Geometry check sheet. Reference: the model listing, model coordinates, mm. Coordinates: 2 decimals unless noted, no trailing zeros. Order: outer loops, then holes, each group sorted by start corner. A loop starts at its lowest first (then second) coordinate and runs counter-clockwise, first axis right, second up. Notation, with made-up numbers: (89.25, -6) - (96.25, -6) arc R13 cw to (96.25, 9) - close; hole circle Ø4 at (-14, 50.25). An arc over 180 degrees is marked (long way). Return JSON: item names as keys, results as strings. Group by question number.
Item 1: Scan lines: probe 1 along Y at (x, z) = (34, -25.1); probe 2 along Y at (x, z) = (104, -25.55); probe 3 along X at (y, z) = (-13, -25.75). Record each from-to range of solid material in increasing order.
Item 2: Draft check along X on faces 1 (the cylindrical face through (-1, 0, -24)), 2 (the cylindrical face through (2.386, 11.425, -24.028)), 3 (the flat face through (51, -30, -24)). Enter one of: pulls with the +X half, pulls with the -X half, needs draft (parallel to the pull), parting line crosses it, or undercut.
Item 3: Section check A-A on y = 0. Enter the section's corners in (x, z).
Item 4: Gauge pin test, flat ends, axial feed: pin 1 (1 mm diameter, centred on x = 9, z = -22.5, fed in from +Y); pin 2 (10.5 mm diameter, centred on x = 16, y = 34, fed in from +Z). Record the tip position at first contact, or that the pin passes through.
Item 5: Section check B-B on z = -25.3. Give the number of separate pieces and of enclosed holes in the cut face, then the cut area to 3 significant figures.
from build123d import *

# Parameters (mm, degrees)
CYLINDER1946_R     = 17
CYLINDER1946_DEPTH = 160
CYLINDER1910_R     = 1.5
CYLINDER1910_DEPTH = 100
CYLINDER1943_R     = 1.5
CYLINDER1943_DEPTH = 100
CYLINDER1944_R     = 1.5
CYLINDER1944_DEPTH = 32
CYLINDER1903_R     = 1.5
CYLINDER1903_DEPTH = 32
BOX555_W           = 200
BOX555_H           = 100
BOX555_DEPTH       = 100
BOX556_W           = 200
BOX556_H           = 100
BOX556_DEPTH       = 100
CYLINDER1907_R     = 4
CYLINDER1907_DEPTH = 100
CYLINDER1908_R     = 4
CYLINDER1908_DEPTH = 100
CYLINDER1912_R     = 4
CYLINDER1912_DEPTH = 100
CYLINDER1913_R     = 4
CYLINDER1913_DEPTH = 100
CYLINDER1914_R     = 4
CYLINDER1914_DEPTH = 100
CYLINDER1901_R     = 4
CYLINDER1901_DEPTH = 100
CYLINDER1902_R     = 4
CYLINDER1902_DEPTH = 100
CYLINDER1919_R     = 4
CYLINDER1919_DEPTH = 100
CYLINDER1927_R     = 1.5
CYLINDER1927_DEPTH = 100
CYLINDER1926_R     = 1.5
CYLINDER1926_DEPTH = 100
CYLINDER1891_R     = 1.5
CYLINDER1891_DEPTH = 100
CYLINDER1894_R     = 1.5
CYLINDER1894_DEPTH = 100
CYLINDER1917_R     = 1.5
CYLINDER1917_DEPTH = 100
CYLINDER1898_R     = 1.5
CYLINDER1898_DEPTH = 100
CYLINDER1920_R     = 1.5
CYLINDER1920_DEPTH = 100
CYLINDER1924_R     = 1.5
CYLINDER1924_DEPTH = 100
CYLINDER1925_R     = 59
CYLINDER1925_DEPTH = 4
FILLET029_R        = 8
FILLET027_R        = 8


with BuildPart() as obj1:
    # Cylinder1946 → Cylinder1946 (new body)
    with BuildSketch(Plane(origin=(-18, 0, -60), x_dir=(1, 0, 0), z_dir=(0, 0, 1))):
        Circle(CYLINDER1946_R)
    extrude(amount=CYLINDER1946_DEPTH)


with BuildPart() as obj2:
    # Cylinder1910 → Cylinder1910 (new body)
    with BuildSketch(Plane(origin=(14, 0, -60), x_dir=(1, 0, 0), z_dir=(0, 0, 1))):
        Circle(CYLINDER1910_R)
    extrude(amount=CYLINDER1910_DEPTH)


with BuildPart() as obj3:
    # Cylinder1943 → Cylinder1943 (new body)
    with BuildSketch(Plane(origin=(90, 0, -60), x_dir=(1, 0, 0), z_dir=(0, 0, 1))):
        Circle(CYLINDER1943_R)
    extrude(amount=CYLINDER1943_DEPTH)

    # Compound988: union obj2
    add(obj2.part)


with BuildPart() as obj4:
    # Cylinder1944 → Cylinder1944 (new body)
    with BuildSketch(Plane(origin=(78, 41, -42), x_dir=(1, 0, 0), z_dir=(0, 0, 1))):
        Circle(CYLINDER1944_R)
    extrude(amount=CYLINDER1944_DEPTH)


with BuildPart() as compound991:
    # Cylinder1903 → Cylinder1903 (new body)
    with BuildSketch(Plane(origin=(26, 41, -42), x_dir=(1, 0, 0), z_dir=(0, 0, 1))):
        Circle(CYLINDER1903_R)
    extrude(amount=CYLINDER1903_DEPTH)

    # Compound991: union obj4
    add(obj4.part)


with BuildPart() as krychle555:
    # Box555 → Box555 (new body)
    with BuildSketch(Plane(origin=(-60, 44, -90), x_dir=(1, 0, 0), z_dir=(0, 0, 1))):
        with Locations((100, 50)):
            Rectangle(BOX555_W, BOX555_H)
    extrude(amount=BOX555_DEPTH)


with BuildPart() as krychle556:
    # Box556 → Box556 (new body)
    with BuildSketch(Plane(origin=(-60, -130, -90), x_dir=(1, 0, 0), z_dir=(0, 0, 1))):
        with Locations((100, 50)):
            Rectangle(BOX556_W, BOX556_H)
    extrude(amount=BOX556_DEPTH)


with BuildPart() as obj5:
    # Cylinder1907 → Cylinder1907 (new body)
    with BuildSketch(Plane(origin=(-16, 34, -90), x_dir=(1, 0, 0), z_dir=(0, 0, 1))):
        Circle(CYLINDER1907_R)
    extrude(amount=CYLINDER1907_DEPTH)


with BuildPart() as obj6:
    # Cylinder1908 → Cylinder1908 (new body)
    with BuildSketch(Plane(origin=(-16, -34, -90), x_dir=(1, 0, 0), z_dir=(0, 0, 1))):
        Circle(CYLINDER1908_R)
    extrude(amount=CYLINDER1908_DEPTH)


with BuildPart() as obj7:
    # Cylinder1912 → Cylinder1912 (new body)
    with BuildSketch(Plane(origin=(34, -16, -90), x_dir=(1, 0, 0), z_dir=(0, 0, 1))):
        Circle(CYLINDER1912_R)
    extrude(amount=CYLINDER1912_DEPTH)


with BuildPart() as obj8:
    # Cylinder1913 → Cylinder1913 (new body)
    with BuildSketch(Plane(origin=(16, 34, -90), x_dir=(1, 0, 0), z_dir=(0, 0, 1))):
        Circle(CYLINDER1913_R)
    extrude(amount=CYLINDER1913_DEPTH)


with BuildPart() as obj9:
    # Cylinder1914 → Cylinder1914 (new body)
    with BuildSketch(Plane(origin=(16, -34, -90), x_dir=(1, 0, 0), z_dir=(0, 0, 1))):
        Circle(CYLINDER1914_R)
    extrude(amount=CYLINDER1914_DEPTH)


with BuildPart() as obj10:
    # Cylinder1901 → Cylinder1901 (new body)
    with BuildSketch(Plane(origin=(-34, 16, -90), x_dir=(1, 0, 0), z_dir=(0, 0, 1))):
        Circle(CYLINDER1901_R)
    extrude(amount=CYLINDER1901_DEPTH)


with BuildPart() as obj11:
    # Cylinder1902 → Cylinder1902 (new body)
    with BuildSketch(Plane(origin=(34, 16, -90), x_dir=(1, 0, 0), z_dir=(0, 0, 1))):
        Circle(CYLINDER1902_R)
    extrude(amount=CYLINDER1902_DEPTH)


with BuildPart() as obj12:
    # Cylinder1919 → Cylinder1919 (new body)
    with BuildSketch(Plane(origin=(-34, -16, -90), x_dir=(1, 0, 0), z_dir=(0, 0, 1))):
        Circle(CYLINDER1919_R)
    extrude(amount=CYLINDER1919_DEPTH)

    # Compound981: union obj5, obj6, obj7, obj8, obj9, obj10, obj11
    add(obj5.part)
    add(obj6.part)
    add(obj7.part)
    add(obj8.part)
    add(obj9.part)
    add(obj10.part)
    add(obj11.part)


with BuildPart() as obj13:
    # Cylinder1927 → Cylinder1927 (new body)
    with BuildSketch(Plane(origin=(103, 12, -60), x_dir=(1, 0, 0), z_dir=(0, 0, 1))):
        Circle(CYLINDER1927_R)
    extrude(amount=CYLINDER1927_DEPTH)


with BuildPart() as obj14:
    # Cylinder1926 → Cylinder1926 (new body)
    with BuildSketch(Plane(origin=(76, 24, -60), x_dir=(1, 0, 0), z_dir=(0, 0, 1))):
        Circle(CYLINDER1926_R)
    extrude(amount=CYLINDER1926_DEPTH)


with BuildPart() as obj15:
    # Cylinder1891 → Cylinder1891 (new body)
    with BuildSketch(Plane(origin=(91, -27, -60), x_dir=(1, 0, 0), z_dir=(0, 0, 1))):
        Circle(CYLINDER1891_R)
    extrude(amount=CYLINDER1891_DEPTH)


with BuildPart() as obj16:
    # Cylinder1894 → Cylinder1894 (new body)
    with BuildSketch(Plane(origin=(13, -27, -60), x_dir=(1, 0, 0), z_dir=(0, 0, 1))):
        Circle(CYLINDER1894_R)
    extrude(amount=CYLINDER1894_DEPTH)


with BuildPart() as obj17:
    # Cylinder1917 → Cylinder1917 (new body)
    with BuildSketch(Plane(origin=(28, 24, -60), x_dir=(1, 0, 0), z_dir=(0, 0, 1))):
        Circle(CYLINDER1917_R)
    extrude(amount=CYLINDER1917_DEPTH)


with BuildPart() as obj18:
    # Cylinder1898 → Cylinder1898 (new body)
    with BuildSketch(Plane(origin=(1, -12, -60), x_dir=(1, 0, 0), z_dir=(0, 0, 1))):
        Circle(CYLINDER1898_R)
    extrude(amount=CYLINDER1898_DEPTH)


with BuildPart() as obj19:
    # Cylinder1920 → Cylinder1920 (new body)
    with BuildSketch(Plane(origin=(1, 12, -60), x_dir=(1, 0, 0), z_dir=(0, 0, 1))):
        Circle(CYLINDER1920_R)
    extrude(amount=CYLINDER1920_DEPTH)


with BuildPart() as obj20:
    # Cylinder1924 → Cylinder1924 (new body)
    with BuildSketch(Plane(origin=(103, -12, -60), x_dir=(1, 0, 0), z_dir=(0, 0, 1))):
        Circle(CYLINDER1924_R)
    extrude(amount=CYLINDER1924_DEPTH)

    # Compound979: union obj13, obj14, obj15, obj16, obj17, obj18, obj19
    add(obj13.part)
    add(obj14.part)
    add(obj15.part)
    add(obj16.part)
    add(obj17.part)
    add(obj18.part)
    add(obj19.part)


with BuildPart() as fillet027:
    # Cylinder1925 → Cylinder1925 (new body)
    with BuildSketch(Plane(origin=(52, 0, -26), x_dir=(1, 0, 0), z_dir=(0, 0, 1))):
        Circle(CYLINDER1925_R)
    extrude(amount=CYLINDER1925_DEPTH)

    # Cut630: cut obj20
    add(obj20.part, mode=Mode.SUBTRACT)

    # Cut644: cut obj12
    add(obj12.part, mode=Mode.SUBTRACT)

    # Cut645: cut Krychle556
    add(krychle556.part, mode=Mode.SUBTRACT)

    # Cut646: cut Krychle555
    add(krychle555.part, mode=Mode.SUBTRACT)

    # Cut647: cut Compound991
    add(compound991.part, mode=Mode.SUBTRACT)

    # Cut651: cut obj3
    add(obj3.part, mode=Mode.SUBTRACT)

    # Cut636: cut obj1
    add(obj1.part, mode=Mode.SUBTRACT)

    # Fillet029
    fillet029_edges = [fillet027.edges().sort_by_distance(p)[0] for p in [
        (-5.8, -11.838919, -24),
    ]]
    fillet(fillet029_edges, radius=FILLET029_R)

    # Fillet027
    fillet027_edges = [fillet027.edges().sort_by_distance(p)[0] for p in [
        (-5.8, 11.838919, -24),
    ]]
    fillet(fillet027_edges, radius=FILLET027_R)


solid = fillet027.part
Computed:
{
 "1": {"probe 1": "y = -30 to -20, -12 to 12, 20 to 44", "probe 2": "y = -27.87 to -13.12, -10.88 to 10.88, 13.12 to 27.87", "probe 3": "x = -5.08 to -0.12, 2.12 to 31.35, 36.65 to 101.88, 104.12 to 109.55"},
 "2": {"face 1": "pulls with the -X half", "face 2": "undercut", "face 3": "needs draft"},
 "3": {"outline": "(-1, -26) - (12.5, -26) - (12.5, -22) - (-1, -22) - close; (15.5, -26) - (88.5, -26) - (88.5, -22) - (15.5, -22) - close; (91.5, -26) - (111, -26) - (111, -22) - (91.5, -22) - close"},
 "4": {"pin 1": "stops at y = 40.92", "pin 2": "stops at z = -22"},
 "5": {"separate pieces": "1", "enclosed holes": "15", "area": "7,700 mm²"}
}
